```python
from build123d import *

# Parameters (mm, degrees)
SKETCH_1_W      = 17
SKETCH_1_H      = 17
EXTRUDE_1_DEPTH = 17
CHAMFER_1_SIZE  = 3.5


with BuildPart() as part:
    # Эскиз1 → Бобышка-Вытянуть1 (new body)
    with BuildSketch(Plane.XY):
        with Locations((8.5, 8.5)):
            Rectangle(SKETCH_1_W, SKETCH_1_H)
    extrude(amount=EXTRUDE_1_DEPTH)

    # Эскиз2 → Отверстие обработанное метчиком M4x0.71 (revolve, cut)
    with BuildSketch(Plane(origin=(11, 17, 13), x_dir=(0, 0, 1), z_dir=(1, 0, 0))):
        Polygon((0, 0), (0, 17), (2.25, 17), (2, 16.75), (2, 0.25), (2.25, 0), align=None)
    revolve(axis=Axis((11, 23.35, 13), (0, -1, 0)), mode=Mode.SUBTRACT)

    # Эскиз2 at point 2 (carried to point 2, square into its face) → Отверстие обработанное метчиком M4x0.71 at 2 (revolve, cut)
    with BuildSketch(Plane(origin=(4, 6, 17), x_dir=(0, -1, 0), z_dir=(1, 0, 0))):
        Polygon((0, 0), (0, 17), (2.25, 17), (2, 16.75), (2, 0.25), (2.25, 0), align=None)
    revolve(axis=Axis((4, 6, 23.35), (0, 0, -1)), mode=Mode.SUBTRACT)

    # Эскиз2 at point 3 (carried to point 3, square into its face) → Отверстие обработанное метчиком M4x0.71 at 3 (revolve, cut)
    with BuildSketch(Plane(origin=(0, 13, 6), x_dir=(0, 0, 1), z_dir=(0, 1, 0))):
        Polygon((0, 0), (0, 17), (2.25, 17), (2, 16.75), (2, 0.25), (2.25, 0), align=None)
    revolve(axis=Axis((-6.35, 13, 6), (1, 0, 0)), mode=Mode.SUBTRACT)

    # Фаска1
    chamfer_1_edges = [part.edges().sort_by_distance(p)[0] for p in [
        (17, 8.5, 0),
        (8.5, 0, 0),
        (17, 0, 8.5),
    ]]
    chamfer(chamfer_1_edges, length=CHAMFER_1_SIZE)


solid = part.part
```
Here's how the part is built. I have some questions about the finished solid (model axes, mm). Coordinates: 2 decimals unless noted, no trailing zeros. Order: outer loops, then holes, each group sorted by start corner. A loop starts at its lowest first (then second) coordinate and runs counter-clockwise, first axis right, second up.
1) Imagine slicing it at A-A on y = 6. List the corners of the cut face in (x, z) for me.
2) I need wall thicknesses on line 1 (X direction, y = 6, z = 13); line 2 (Z direction, x = 4, y = 13); line 3 (Y direction, x = 4, z = 5.5). Which ranges of each line are inside material? Lowest first, please.
3) Imagine slicing it at D-D on y = 2. List the corners of the cut face in (x, z) for me, and give its area (3 significant figures).
4) Imagine slicing it at B-B on z = 6. List the corners of the cut face in (x, y) for me.
5) Imagine slicing it at C-C on x = 13.75. List the corners of the cut face in (y, z) for me, and give its area (3 significant figures).
6) We'd pull the mould along X, two halves only. Please class faces 1 (the face through (8, 9, 17)), 2 (the face through (5.2, 7.6, 8.6)), 3 (the face through (17, 10, 10)): +X half, -X half, draft (parallel to the pull), parting line (faces both ways), or undercut.
7) Will this pin go through, and if not, where does the flat tip stop? pin 1 (3 mm diameter, centred on x = 3.5, y = 6.5, fed in from -Z).
Response values:
1. outline: (0, 0) - (1.75, 0) - (2, 0.25) - (2, 16.75) - (1.75, 17) - (0, 17) - close; (6, 0.25) - (6.25, 0) - (13.5, 0) - (17, 3.5) - (17, 17) - (6.25, 17) - (6, 16.75) - close; hole circle Ø4 at (11, 13)
2. line 1: x = 0 to 2, 6 to 9, 13 to 17
2. line 2: z = 0 to 4, 8 to 17
2. line 3: y = 0 to 4, 8 to 11.06, 14.94 to 17
3. outline: (0, 1.5) - (13.5, 1.5) - (15.5, 3.5) - (15.5, 17) - (0, 17) - close; hole circle Ø4 at (11, 13)
3. area: 226 mm2
4. outline: (0, 0) - (13.5, 0) - (17, 3.5) - (17, 10.75) - (16.75, 11) - (0.25, 11) - (0, 10.75) - close; (0, 15.25) - (0.25, 15) - (16.75, 15) - (17, 15.25) - (17, 17) - (0, 17) - close; hole circle Ø4 at (4, 6)
5. outline: (0.25, 3.5) - (3.5, 0.25) - (17, 0.25) - (17, 17) - (0.25, 17) - close; hole circle Ø4 at (13, 6)
5. area: 263 mm2
6. face 1: draft
6. face 2: undercut
6. face 3: +X half
7. pin 1: stops at z = 0.04
